Could you check a few things on this drawing? It's one solid part, dimensions in mm from its lowest x, y, z. Give positions to 0.01 mm unless a question says otherwise; leave off trailing zeros. Order: outer loops, then holes, each group sorted by start corner. A loop starts at its lowest first (then second) coordinate and runs counter-clockwise, first axis right, second up.
Item 1: I want a section at A-A, the plane y = 17.5. Write out the boundary of the cut face in (x, z).
Item 2: I want a section at D-D, the plane z = 2.5. Write out the boundary of the cut face in (x, y), then the cut area to 3 significant figures.
Item 3: I'm going to push flat-ended pins straight in: pin 1 Ø6 at (x, z) = (89, 6.5) entering from -Y; pin 2 Ø10 at (x, z) = (11, 2.5) entering from -Y; pin 3 Ø8 at (x, z) = (42, 3.5) entering from +Y. Where does each tip first touch, or does it pass through?
Item 4: I want a section at B-B, the plane x = 85. Write out the boundary of the cut face in (y, z).
Item 5: I want a section at C-C, the plane z = 12.5. Write out the boundary of the cut face in (x, y).
Item 6: If we mould it in two halves opening along X, with no side actions, what happens to the marked faces 1, 2 and 3? For each: +X half, -X half, draft (parallel to the pull), parting line (faces both ways), or undercut.
Item 7: If I drill on line 1 along X through (y, z) = (17.5, 10); line 2 along X through (y, z) = (19, 7.75); line 3 along Y through (x, z) = (85, 14.5), over which ranges is the centre line in solid material (lowest first)?
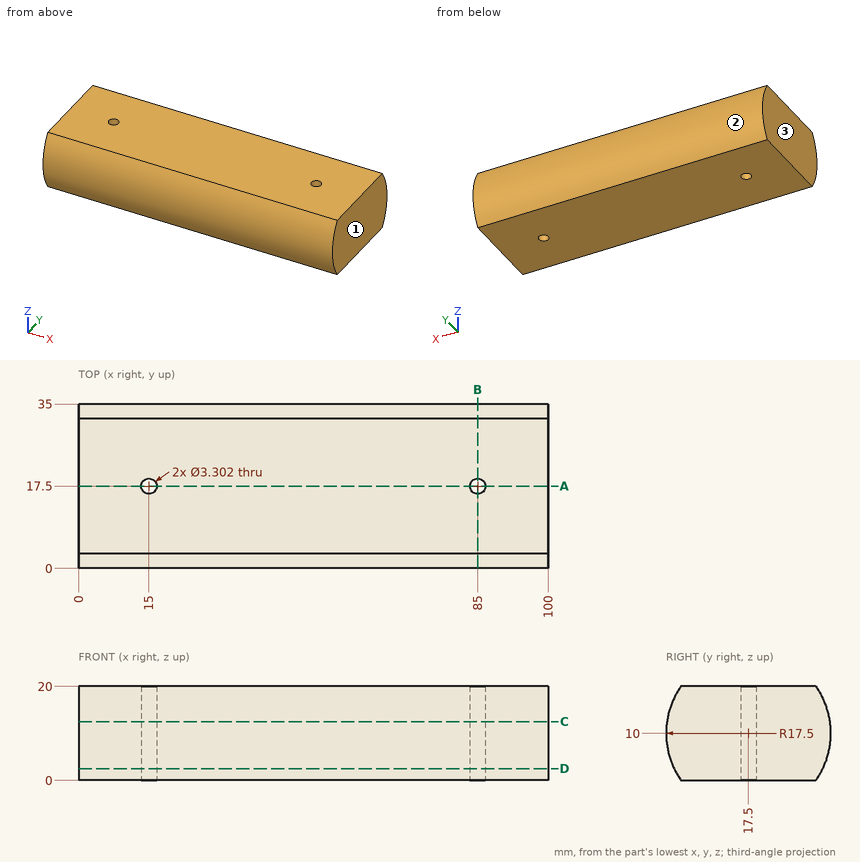
Results list:
1. outline: (0, 0) - (13.35, 0) - (13.35, 20) - (0, 20) - close; (16.65, 0) - (83.35, 0) - (83.35, 20) - (16.65, 20) - close; (86.65, 0) - (100, 0) - (100, 20) - (86.65, 20) - close
2. outline: (0, 1.69) - (100, 1.69) - (100, 33.31) - (0, 33.31) - close; hole circle Ø3.3 at (15, 17.5); hole circle Ø3.3 at (85, 17.5)
2. area: 3,150 mm2
3. pin 1: stops at y = 0.01
3. pin 2: stops at y = 0.18
3. pin 3: stops at y = 34.82
4. outline: (3.14, 0) - (15.85, 0) - (15.85, 20) - (3.14, 20) arc R17.5 ccw to start; (19.15, 0) - (31.86, 0) arc R17.5 ccw to (31.86, 20) - (19.15, 20) - close
5. outline: (0, 0.18) - (100, 0.18) - (100, 34.82) - (0, 34.82) - close; hole circle Ø3.3 at (15, 17.5); hole circle Ø3.3 at (85, 17.5)
6. face 1: +X half
6. face 2: draft
6. face 3: -X half
7. line 1: x = 0 to 13.35, 16.65 to 83.35, 86.65 to 100
7. line 2: x = 0 to 14.31, 15.69 to 84.31, 85.69 to 100
7. line 3: y = 0.59 to 15.85, 19.15 to 34.41
